```python
from build123d import *

# Parameters (mm, degrees)
SKETCH_1_W           = 60
SKETCH_1_H           = 34
EXTRUDE_1_DEPTH      = 30
SKETCH_17_W          = 12
SKETCH_17_H          = 23
EXTRUDE_8_DEPTH      = 80
SKETCH_18_R          = 2
CUT_EXTRUDE_7_DEPTH  = 10
CUT_EXTRUDE_8_DEPTH  = 66
SKETCH_20_W          = 4.5
SKETCH_20_H          = 17.2
CUT_EXTRUDE_9_DEPTH  = 8.8
SKETCH_14_R          = 1.6
CUT_EXTRUDE_6_DEPTH  = 103.708324882
EXTRUDE_START        = 7
SKETCH_21_W          = 60
SKETCH_21_H          = 30
SKETCH_21_R          = 1.6
EXTRUDE_9_DEPTH      = 7
SKETCH_22_W          = 36
SKETCH_22_H          = 30
EXTRUDE_10_DEPTH     = 7
SKETCH_27_W          = 12
SKETCH_27_H          = 50
CUT_EXTRUDE_13_DEPTH = 95.768138106
SKETCH_29_W          = 12
SKETCH_29_H          = 16
CUT_EXTRUDE_14_DEPTH = 71.710678119
SKETCH_36_W          = 12
SKETCH_36_H          = 23
CUT_EXTRUDE_21_DEPTH = 50
SKETCH_37_W          = 12
SKETCH_37_H          = 16
CUT_EXTRUDE_22_DEPTH = 59.309518948
SKETCH_38_W          = 60
SKETCH_38_H          = 30
CUT_EXTRUDE_23_DEPTH = 34
SKETCH_41_W          = 6.9
SKETCH_41_H          = 4.95
SKETCH_41_W_2        = 5.41
SKETCH_41_H_2        = 4.05
CUT_EXTRUDE_25_DEPTH = 5.5
CUT_EXTRUDE_26_DEPTH = 49.744230428
SKETCH_43_R          = 1.35
CUT_EXTRUDE_27_DEPTH = 49.7442306
SKETCH_47_R          = 1.9
CUT_EXTRUDE_29_DEPTH = 7
SKETCH_48_R          = 2
CUT_EXTRUDE_30_DEPTH = 10
CUT_EXTRUDE_START    = -4
SKETCH_49_R          = 2
CUT_EXTRUDE_31_DEPTH = 4.9
CUT_EXTRUDE_32_DEPTH = 4.05
CUT_EXTRUDE_33_DEPTH = 4.95
CUT_EXTRUDE_34_REACH = 50.744
SKETCH_53_R          = 2


with BuildPart() as part:
    # 草图1 → 凸台-拉伸1 (new body)
    with BuildSketch(Plane.XY):
        Rectangle(SKETCH_1_W, SKETCH_1_H)
    extrude(amount=EXTRUDE_1_DEPTH)

    # 草图17 → 凸台-拉伸8 (add)
    with BuildSketch(Plane(origin=(0, 0, 0), x_dir=(-1, 0, 0), z_dir=(0, 0, -1))):
        with Locations((24, 28.5)):
            Rectangle(SKETCH_17_W, SKETCH_17_H)
        with Locations((-24, 28.5)):
            Rectangle(SKETCH_17_W, SKETCH_17_H)
    extrude(amount=-EXTRUDE_8_DEPTH)

    # 草图18 → 切除-拉伸7 (cut)
    with BuildSketch(Plane.XY.offset(80)):
        with Locations((24.5, 34)):
            Circle(SKETCH_18_R)
        with Locations((24.5, 24)):
            Circle(SKETCH_18_R)
        with Locations((-24.5, 24)):
            Circle(SKETCH_18_R)
        with Locations((-24.5, 34)):
            Circle(SKETCH_18_R)
    extrude(amount=-CUT_EXTRUDE_7_DEPTH, mode=Mode.SUBTRACT)

    # 草图19 → 切除-拉伸8 (cut)
    with BuildSketch(Plane.XY.offset(30)):
        with BuildLine():
            Line((2, 12.4), (-6, 12.4))
            ThreePointArc((-6, 12.4), (-15.249310993, 0), (-6, -12.4))
            Line((-6, -12.4), (2, -12.4))
            Line((2, -12.4), (16.003706397, -7.024480757))
            ThreePointArc((16.003706397, -7.024480757), (17.250689007, 0), (16.003706397, 7.024480757))
            Line((16.003706397, 7.024480757), (2, 12.4))
        make_face()
    extrude(amount=-CUT_EXTRUDE_8_DEPTH, mode=Mode.SUBTRACT)

    # 草图20 → 切除-拉伸9 (cut)
    with BuildSketch(Plane(origin=(30, 0, 0), x_dir=(0, 0, -1), z_dir=(1, 0, 0))):
        with Locations((-67.75, 28.8)):
            Rectangle(SKETCH_20_W, SKETCH_20_H)
    cut_extrude_9 = extrude(amount=-CUT_EXTRUDE_9_DEPTH, mode=Mode.SUBTRACT)

    # 草图14 → 切除-拉伸6 (cut, through all)
    with BuildSketch(Plane.XZ.offset(17)):
        with Locations(Location((24.5, 15, 0), (0, 0, 270))):
            Circle(SKETCH_14_R)
        with Locations(Location((-24.5, 15, 0), (0, 0, 270))):
            Circle(SKETCH_14_R)
    extrude(amount=-CUT_EXTRUDE_6_DEPTH, mode=Mode.SUBTRACT)

    # 镜向3: 切除-拉伸9 across plane
    add(cut_extrude_9.mirror(Plane(origin=(0, 0, 0), x_dir=(0, 0, 1), z_dir=(1, 0, 0))), mode=Mode.SUBTRACT)

    # 草图21 → 凸台-拉伸9 (add)
    with BuildSketch(Plane.XZ.offset(17).offset(EXTRUDE_START)):
        with Locations((0, 15)):
            Rectangle(SKETCH_21_W, SKETCH_21_H)
        with Locations(Location((24.5, 15, 0), (0, 0, 270))):
            Circle(SKETCH_21_R, mode=Mode.SUBTRACT)
        with Locations(Location((-24.5, 15, 0), (0, 0, 270))):
            Circle(SKETCH_21_R, mode=Mode.SUBTRACT)
    extrude(amount=-EXTRUDE_9_DEPTH)

    # 草图22 → 凸台-拉伸10 (add)
    with BuildSketch(Plane(origin=(0, 17, 0), x_dir=(1, 0, 0), z_dir=(0, 1, 0))):
        with Locations((0, -15)):
            Rectangle(SKETCH_22_W, SKETCH_22_H)
    extrude(amount=EXTRUDE_10_DEPTH)

    # 草图27 → 切除-拉伸13 (cut, through all)
    with BuildSketch(Plane.XZ.offset(-17)):
        with Locations((24, 55)):
            Rectangle(SKETCH_27_W, SKETCH_27_H)
    extrude(amount=-CUT_EXTRUDE_13_DEPTH, mode=Mode.SUBTRACT)

    # 草图29 → 切除-拉伸14 (cut, through all)
    with BuildSketch(Plane.XY.offset(30)):
        with Locations((24, 32)):
            Rectangle(SKETCH_29_W, SKETCH_29_H)
    extrude(amount=-CUT_EXTRUDE_14_DEPTH, mode=Mode.SUBTRACT)

    # 草图36 → 切除-拉伸21 (cut)
    with BuildSketch(Plane.XY.offset(80)):
        with Locations((-24, 28.5)):
            Rectangle(SKETCH_36_W, SKETCH_36_H)
    extrude(amount=-CUT_EXTRUDE_21_DEPTH, mode=Mode.SUBTRACT)

    # 草图37 → 切除-拉伸22 (cut, through all)
    with BuildSketch(Plane.XY.offset(30)):
        with Locations((-24, 32)):
            Rectangle(SKETCH_37_W, SKETCH_37_H)
    extrude(amount=-CUT_EXTRUDE_22_DEPTH, mode=Mode.SUBTRACT)

    # 草图38 → 切除-拉伸23 (cut)
    with BuildSketch(Plane(origin=(0, 0, 0), x_dir=(1, 0, 0), z_dir=(0, 1, 0))):
        with Locations((0, -15)):
            Rectangle(SKETCH_38_W, SKETCH_38_H)
    extrude(amount=-CUT_EXTRUDE_23_DEPTH, mode=Mode.SUBTRACT)

    # 草图41 → 切除-拉伸25 (cut)
    with BuildSketch(Plane(origin=(30, 0, 0), x_dir=(0, 0, -1), z_dir=(1, 0, 0))):
        with Locations((-15, 17.525)):
            Rectangle(SKETCH_41_W, SKETCH_41_H)
        with Locations((-15, 6.025)):
            Rectangle(SKETCH_41_W_2, SKETCH_41_H_2)
    cut_extrude_25 = extrude(amount=-CUT_EXTRUDE_25_DEPTH, mode=Mode.SUBTRACT)

    # 镜向5: 切除-拉伸25 across plane
    add(cut_extrude_25.mirror(Plane(origin=(0, 0, 0), x_dir=(0, 0, 1), z_dir=(1, 0, 0))), mode=Mode.SUBTRACT)

    # 草图42 → 切除-拉伸26 (cut, through all)
    with BuildSketch(Plane.XY.offset(30)):
        with BuildLine():
            Line((16.003706397, 7.024480757), (14.503027832, 1.394480604))
            Line((14.503027832, 1.394480604), (17.250689007, 0))
            add(Edge.make_bspline(
                [(16.44131127, 6.418576517), (17.679905774, 3.26163083), (17.250689007, 0)],
                knots=[0, 0, 0, 1, 1, 1], degree=2))
            Line((16.44131127, 6.418576517), (16.003706397, 7.024480757))
        make_face()
    extrude(amount=-CUT_EXTRUDE_26_DEPTH, mode=Mode.SUBTRACT)

    # 草图43 → 切除-拉伸27 (cut, through all)
    with BuildSketch(Plane(origin=(0, 24, 0), x_dir=(1, 0, 0), z_dir=(0, 1, 0))):
        with Locations(Location((0, -6, 0), (0, 0, 270))):
            Circle(SKETCH_43_R)
        with Locations(Location((0, -24, 0), (0, 0, 180))):
            Circle(SKETCH_43_R)
    extrude(amount=-CUT_EXTRUDE_27_DEPTH, mode=Mode.SUBTRACT)

    # 草图47 → 切除-拉伸29 (cut)
    with BuildSketch(Plane(origin=(0, 24, 0), x_dir=(1, 0, 0), z_dir=(0, 1, 0))):
        with Locations(Location((-24.5, -15, 0), (0, 0, 270))):
            Circle(SKETCH_47_R)
        with Locations(Location((24.5, -15, 0), (0, 0, 270))):
            Circle(SKETCH_47_R)
    extrude(amount=-CUT_EXTRUDE_29_DEPTH, mode=Mode.SUBTRACT)

    # 草图48 → 切除-拉伸30 (cut)
    with BuildSketch(Plane(origin=(0, 24, 0), x_dir=(1, 0, 0), z_dir=(0, 1, 0))):
        with Locations(Location((-24.5, -5, 0), (0, 0, 270))):
            Circle(SKETCH_48_R)
        with Locations(Location((24.5, -5, 0), (0, 0, 90))):
            Circle(SKETCH_48_R)
    extrude(amount=-CUT_EXTRUDE_30_DEPTH, mode=Mode.SUBTRACT)

    # 草图49 → 切除-拉伸31 (cut)
    # profile 1 of 2: a face of its own
    with BuildSketch(Plane(origin=(0, 24, 0), x_dir=(1, 0, 0), z_dir=(0, 1, 0)).offset(CUT_EXTRUDE_START)):
        Polygon((-26.491858429, -8.45), (-22.508141571, -8.45), (-20.516283143, -5), (-22.508141571, -1.55), (-26.491858429, -1.55), (-28.483716857, -5), align=None)
        with Locations(Location((-24.5, -5, 0), (0, 0, 270))):
            Circle(SKETCH_49_R, mode=Mode.SUBTRACT)
    # profile 2 of 2: a face of its own
    with BuildSketch(Plane(origin=(0, 24, 0), x_dir=(1, 0, 0), z_dir=(0, 1, 0)).offset(CUT_EXTRUDE_START)):
        Polygon((-28.483716857, 0), (-28.483716857, -5), (-26.491858429, -1.55), (-22.508141571, -1.55), (-20.516283143, -5), (-20.516283143, 0), align=None)
    cut_extrude_31 = extrude(amount=-CUT_EXTRUDE_31_DEPTH, mode=Mode.SUBTRACT)

    # 镜向6: 切除-拉伸31 across plane
    add(cut_extrude_31.mirror(Plane(origin=(0, 0, 0), x_dir=(0, 0, 1), z_dir=(1, 0, 0))), mode=Mode.SUBTRACT)

    # 草图51 → 切除-拉伸32 (cut)
    with BuildSketch(Plane.XZ.offset(-8.05)):
        Polygon((26.061732478, 17.705), (22.938267522, 17.705), (21.376535044, 15), (22.938267522, 12.295), (26.061732478, 12.295), (27.623464956, 15), align=None)
    cut_extrude_32 = extrude(amount=CUT_EXTRUDE_32_DEPTH, mode=Mode.SUBTRACT)

    # 草图52 → 切除-拉伸33 (cut)
    with BuildSketch(Plane(origin=(0, 15.05, 0), x_dir=(1, 0, 0), z_dir=(0, 1, 0))):
        Polygon((26.491858429, -11.55), (22.508141571, -11.55), (20.516283143, -15), (22.508141571, -18.45), (26.491858429, -18.45), (28.483716857, -15), align=None)
    cut_extrude_33 = extrude(amount=CUT_EXTRUDE_33_DEPTH, mode=Mode.SUBTRACT)

    # 镜向7: 切除-拉伸32, 切除-拉伸33 across plane
    add(cut_extrude_32.mirror(Plane(origin=(0, 0, 0), x_dir=(0, 0, 1), z_dir=(1, 0, 0))), mode=Mode.SUBTRACT)
    add(cut_extrude_33.mirror(Plane(origin=(0, 0, 0), x_dir=(0, 0, 1), z_dir=(1, 0, 0))), mode=Mode.SUBTRACT)

    # 草图53 → 切除-拉伸34 (cut, up to next)
    with BuildSketch(Plane(origin=(0, 24, 0), x_dir=(1, 0, 0), z_dir=(0, 1, 0)), mode=Mode.PRIVATE) as cut_extrude_34_sk1:
        with Locations(Location((-24.5, -15, 0), (0, 0, 270))):
            Circle(SKETCH_53_R)
    cut_extrude_34_tool1 = extrude(cut_extrude_34_sk1.sketch, amount=-CUT_EXTRUDE_34_REACH, mode=Mode.PRIVATE) & part.part
    # 草图53 → 切除-拉伸34 (cut, up to next)
    with BuildSketch(Plane(origin=(0, 24, 0), x_dir=(1, 0, 0), z_dir=(0, 1, 0)), mode=Mode.PRIVATE) as cut_extrude_34_sk2:
        with Locations(Location((24.5, -15, 0), (0, 0, 270))):
            Circle(SKETCH_53_R)
    cut_extrude_34_tool2 = extrude(cut_extrude_34_sk2.sketch, amount=-CUT_EXTRUDE_34_REACH, mode=Mode.PRIVATE) & part.part
    add(cut_extrude_34_tool1.solids().sort_by_distance((-24.5, 24, 15))[0], mode=Mode.SUBTRACT)
    add(cut_extrude_34_tool1.solids().sort_by_distance((-24.5, 24, 15))[1], mode=Mode.SUBTRACT)
    add(cut_extrude_34_tool2.solids().sort_by_distance((24.5, 24, 15))[0], mode=Mode.SUBTRACT)
    add(cut_extrude_34_tool2.solids().sort_by_distance((24.5, 24, 15))[1], mode=Mode.SUBTRACT)


solid = part.part
```
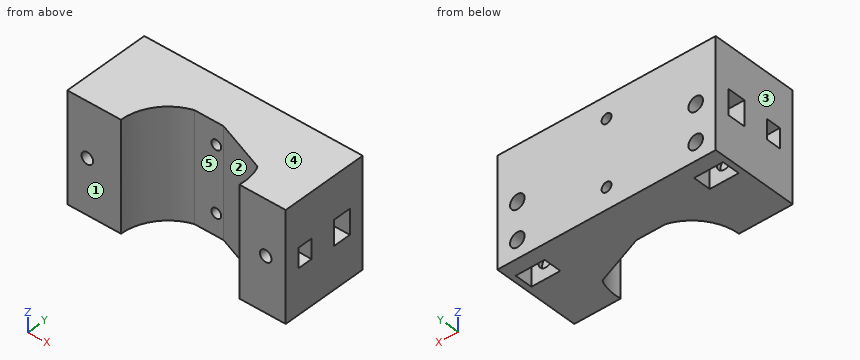
CAD build for the part. Positions are in the model's coordinates, mm. Face numbers are marked on the shaded views. A direction names the side the tool comes from. Round coordinates to 2 decimals unless told otherwise and drop trailing zeros. Order: outer loops, then holes, each group sorted by start corner. A loop starts at its lowest first (then second) coordinate and runs counter-clockwise, first axis right, second up. Notation, with made-up numbers: (-29.5, 27.25) - (-8.5, 27.25) arc R17 ccw to (-8.5, 58.25) - close; hole circle Ø11 at (-39.5, 64). An arc over 180 degrees is marked (long way). Answer as CSV lines item,"result". Start each with the question number.
1. Pull direction X, two halves, no side cores. Call the marked faces 1, 2 and 3: +X half, -X half, draft (parallel to the pull), parting line (faces both ways), or undercut.
2. Saw through at B-B, the plane x = -14. Write the cut outline in (y, z), and give its area (3 significant figures).
3. Pin check, flat tips, straight feed: pin 1 (5 mm diameter, centred on x = 13.5, y = 4, fed in from -Z); pin 2 (4 mm diameter, centred on x = -23.5, y = 17.5, fed in from -Z); pin 3 (3.5 mm diameter, centred on x = -24.5, z = 15, fed in from +Y); pin 4 (5 mm diameter, centred on x = 13, z = 8, fed in from -Y). Stop position of each tip, or through.
4. Tool access for the marked faces 4 and 5: list every direction of +Z, -Z, +X, -X, +Y, -Y with a clear straight run to the whole face (end or side of a thin tool).
5. Drill centre lines: L1, parallel to Y at x = 26.5, z = 15.5; L2, parallel to Z at x = 24.5, y = 3.2; L3, parallel to X at y = 22.5, z = 15. Where is each one in solid material? Low to high. Write a range as [from, to].
6. Saw through at A-A, the plane x = 24.5. Count the separate pieces of the cut face and the enclosed holes in it, and give its area (3 significant figures).
Model answer:
1,face 1,"draft"
1,face 2,"undercut"
1,face 3,"-X half"
2,outline,"(5.55, 0) - (24, 0) - (24, 30) - (5.55, 30) - close"
2,area,"554 mm²"
3,pin 1,"passes through"
3,pin 2,"stops at z = 6.7"
3,pin 3,"stops at y = 4"
3,pin 4,"stops at y = 7.22"
4,face 4,"+Z, +X, -X, +Y, -Y"
4,face 5,"+Z, -Z, -Y"
5,L1,"y = [0, 4], [8.05, 15.05], [20, 24]"
5,L2,"z = [0, 13.4], [16.6, 30]"
5,L3,"x = [-30, -26.5], [-22.5, 22.5], [26.5, 30]"
6,separate pieces,"3"
6,enclosed holes,"0"
6,area,"545 mm²"
